```python
from build123d import *


with BuildPart() as f1:
    # F0 (on Front) → F1 (revolve)
    with BuildSketch(Plane.XZ):
        Polygon((0, 32), (0, 0), (80, 0), (80, 84), (76.87731, 84), (75.5, 80), (71.368069, 68), (68.631931, 68), (64.5, 80), (63.12269, 84), (62.5, 84), (62.5, 74), (61.87731, 74), (60.5, 70), (56.368069, 58), (53.631931, 58), (49.5, 70), (48.12269, 74), (47.5, 74), (47.5, 60), (46.87731, 60), (45.5, 56), (41.368069, 44), (38.631931, 44), (34.5, 56), (33.12269, 60), (32.5, 60), (32.5, 44), (31.799679, 44), (30.5, 40), (26.600964, 28), (23.399036, 28), (19.5, 40), (18.200321, 44), (17.5, 44), (17.5, 32), (16.722923, 32), (15.5, 28), (11.831232, 16), (8.168768, 16), (4.5, 28), (3.277077, 32), align=None)
    revolve(axis=Axis((40, 0, 0), (1, 0, 0)))


solid = f1.part
```
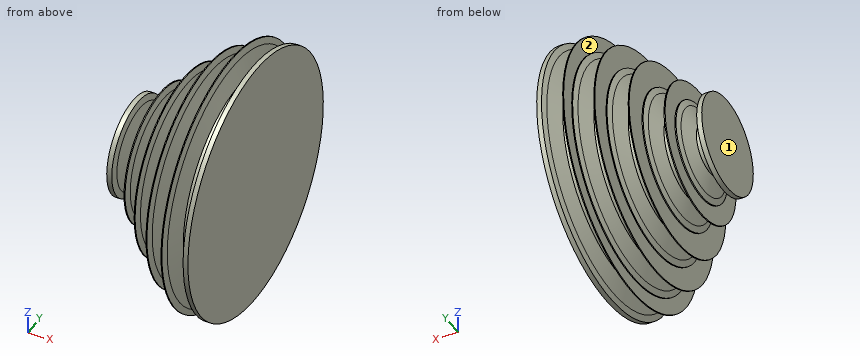
Design review of the part built by this model. Coordinates are the model's own, in mm. Face numbers are marked on the shaded views. A direction names the side the tool comes from. Coordinates: 2 decimals unless noted, no trailing zeros. Answer as a JSON object with one key per item and string values. Group by question number.
1) Wall thickness on L1, parallel to X at y = -50.5, z = -52.5; L2, parallel to X at y = -42, z = -66; L3, parallel to Z at x = 33, y = 15.5: over which ranges is each line inside the solid? List them lowest first.
2) Tool access review of the marked faces 1 and 2: name each direction out of +Z, -Z, +X, -X, +Y, -Y from which nothing blocks a thin tool from reaching the whole face with its end or side.
3) For pin 1 (10 mm diameter, centred on x = 18.5, z = -1, fed in from -Y); pin 2 (12 mm diameter, centred on x = 56, z = 14, fed in from +Y); pin 3 (8 mm diameter, centred on y = 38, z = -62, fed in from -X), all flat-tipped, find the tip position at first contact; note any pin that passes through.
Computed values:
{
 "1": {"L1": "x = 47.5 to 48.52, 61.48 to 66.96, 73.04 to 80", "L2": "x = 62.5 to 65.11, 74.89 to 80", "L3": "z = -57.96 to 57.96"},
 "2": {"face 1": "+Z, -Z, -X, +Y, -Y", "face 2": "-X"},
 "3": {"pin 1": "stops at y = -44", "pin 2": "stops at y = 72.89", "pin 3": "stops at x = 47.5"}
}
